Geometry: final body of the model. Coordinates: model frame, mm. A direction names the side the tool comes from. Round coordinates to 2 decimals unless told otherwise and drop trailing zeros. Order: outer loops, then holes, each group sorted by start corner. A loop starts at its lowest first (then second) coordinate and runs counter-clockwise, first axis right, second up. Notation, with made-up numbers: (-5, 76.5) -> (25, 76.5) arc R16 ccw to (25, 94.5) -> close; hole circle Ø8 at (86, 1). An arc over 180 degrees is marked (long way). Put each result on its own line as item: value.
```python
from build123d import *

# Parameters (mm, degrees)
SKETCH_27_R      = 5
EXTRUDE_14_DEPTH = 60
CHAMFER_2_SIZE   = 5
SKETCH_29_R      = 2
EXTRUDE_15_DEPTH = 17


with BuildPart() as part:
    # 草图27 → 凸台-拉伸14 (new body)
    with BuildSketch(Plane.XY):
        Circle(SKETCH_27_R)
    extrude(amount=EXTRUDE_14_DEPTH)

    # 倒角2
    chamfer_2_edges = [part.edges().sort_by_distance(p)[0] for p in [
        (-5, 0, 60),
    ]]
    chamfer(chamfer_2_edges, length=CHAMFER_2_SIZE)

    # 草图29 → 凸台-拉伸15 (add, symmetric)
    with BuildSketch(Plane(origin=(0, 0, 0), x_dir=(0, 0, -1), z_dir=(1, 0, 0))):
        with Locations((-30.18471694, 0)):
            Circle(SKETCH_29_R)
    extrude(amount=EXTRUDE_15_DEPTH, both=True)


solid = part.part
```
1. Set-up query: faces 5 (the face through (10.878, 0.088, 32.183)), 6 (the face through (17, 0, 30)). Return all of +Z, -Z, +X, -X, +Y, -Y with unobstructed straight access to the full face (end or side cutting, diameter ignored); none if empty.
Ans:
face 5: +X
face 6: +Z, -Z, +X, +Y, -Y
2. Cut plane B-B on x = 12. Return loops of the section in (y, z), and give its area (3 significant figures).
Ans:
outline: circle Ø4 at (0, 30.18)
area: 12.6 mm²
3. Material intervals for probe 1 along X at (y, z) = (2.5, 3); probe 2 along X at (y, z) = (4.5, 7.5); probe 3 along Z at (x, y) = (10, -1.75), sorted ascending.
Ans:
probe 1: -4.33 to 4.33
probe 2: -2.18 to 2.18
probe 3: 29.22 to 31.15
4. Contact query for flat-ended pins moving along their axis: P1, Ø1.5, axis at x = -6, z = 54, coming from the +Y side; P2, Ø4, axis at y = 0, z = 48, coming from the -X side; P3, Ø3, axis at x = 12, y = -1, coming from the -Z side; P4, Ø4, axis at x = -5, z = 33.5, coming from the -Y side. Output: stop coordinate, or through.
Ans:
P1: through
P2: x = -5
P3: z = 28.18
P4: y = -4
5. Draft query along Z for faces 1 (the face through (-10.704, 0.088, 32.183)), 2 (the face through (0, 1, 59)), 3 (the face through (0, 0, 0)), 4 (the face through (-1.08, -4.88, 27.12)). Return one class per face: +Z half, -Z half, draft (parallel to the pull), parting line (faces both ways), or undercut.
Ans:
face 1: parting line
face 2: +Z half
face 3: -Z half
face 4: draft
6. Cut plane A-A on z = 7. Return loops of the section in (x, y), and give its area (3 significant figures).
Ans:
outline: circle Ø10 at (0, 0)
area: 78.5 mm²
